Input: part model. Units: mm. Frame: model coordinates. Give positions to 0.01 mm unless a question says otherwise; leave off trailing zeros. Loops run counter-clockwise (first coordinate to the right, second up) from the corner with the lowest first, then second, coordinate; pieces in that order, holes last. Notation, with made-up numbers: (45.5, 47) - (95.5, 47) arc R20 ccw to (95.5, 86) - close; hole circle Ø7 at (58, -34). An arc over 180 degrees is marked (long way). Answer as a JSON object with one key per item and string values.
from build123d import *

# Parameters (mm, degrees)
SKETCH1_R      = 0.6604
EXTRUDE1_DEPTH = 0.5334
FILLET1_R      = 1.1684


with BuildPart() as part:
    # Sketch1 → Extrude1 (new body, symmetric)
    with BuildSketch(Plane(origin=(0, 0, 0), x_dir=(0, 0, -1), z_dir=(1, 0, 0))):
        with BuildLine():
            Line((-0.179532905, 10.28543324), (-0.240263789, 13.76470325))
            Line((-0.240263789, 13.76470325), (-2.849716296, 13.719155087))
            Line((-2.849716296, 13.719155087), (-4.681521945, 10.760524305))
            ThreePointArc((-4.681521945, 10.760524305), (0, -12.9286), (4.681521945, 10.760524305))
            Line((4.681521945, 10.760524305), (2.849716296, 13.719155087))
            Line((2.849716296, 13.719155087), (0.240263789, 13.76470325))
            Line((0.240263789, 13.76470325), (0.179532905, 10.28543324))
            ThreePointArc((0.179532905, 10.28543324), (0, -10.287), (-0.179532905, 10.28543324))
        make_face()
        with Locations((-1.514624601, 12.002294163)):
            Circle(SKETCH1_R, mode=Mode.SUBTRACT)
        with Locations((1.514624601, 12.002294163)):
            Circle(SKETCH1_R, mode=Mode.SUBTRACT)
    extrude(amount=EXTRUDE1_DEPTH, both=True)

    # Fillet1
    fillet1_edges = [part.edges().sort_by_distance(p)[0] for p in [
        (0, 13.719155087, -2.849716296),
        (0, 10.760524305, -4.681521945),
        (0, 10.760524305, 4.681521945),
        (0, 13.719155087, 2.849716296),
    ]]
    fillet(fillet1_edges, radius=FILLET1_R)


solid = part.part
Item 1: Mould query, pull axis Y, two halves, no side actions, for faces 1 (the face through (0.533, -10.4, 1)), 2 (the face through (-0.01, 11.36, 1.66)), 3 (the face through (0.007, 12.14, 3.827)). Classes: released by +Y, released by -Y, zero draft, split by the parting line, or undercut.
Geometry check:
{"face 1": "zero draft", "face 2": "undercut", "face 3": "released by +Y"}
Item 2: Cut plane B-B (z = -1.5). Return loops of the section in (x, y).
Geometry check:
{"outline": "(-0.53, -12.84) - (0.53, -12.84) - (0.53, -10.18) - (-0.53, -10.18) - close; (-0.53, 10.18) - (0.53, 10.18) - (0.53, 11.34) - (-0.53, 11.34) - close; (-0.53, 12.66) - (0.53, 12.66) - (0.53, 13.74) - (-0.53, 13.74) - close"}
Item 3: Cut plane D-D (z = 9.5). Return loops of the section in (x, y), then the cut area to 3 significant figures.
Geometry check:
{"outline": "(-0.53, -8.45) - (0.53, -8.45) - (0.53, -3.95) - (-0.53, -3.95) - close; (-0.53, 3.95) - (0.53, 3.95) - (0.53, 7.2) - (-0.53, 7.2) - close", "area": "8.27 mm2"}
Item 4: Material intervals for line 1 (Y direction, x = 0.5, z = -2) (3 decimals); line 2 (Y direction, x = -0.05, z = 1); line 3 (Z direction, x = -0.05, y = 4.75), sorted ascending. Write a range as [from, to].
Geometry check:
{"line 1": "y = [-12.765, -10.091], [10.091, 11.554], [12.45, 13.734]", "line 2": "y = [-12.89, -10.24], [10.24, 11.59], [12.42, 13.75]", "line 3": "z = [-11.07, -9.12], [9.12, 11.07]"}
Item 5: Cut plane A-A (y = -0.5). Return loops of the section in (x, z), then the cut area to 3 significant figures.
Geometry check:
{"outline": "(-0.53, -12.31) - (0.53, -12.31) - (0.53, -10.27) - (-0.53, -10.27) - close; (-0.53, 10.27) - (0.53, 10.27) - (0.53, 12.31) - (-0.53, 12.31) - close", "area": "4.33 mm2"}
Item 6: Cut plane C-C (x = 0.15). Return loops of the section in (y, z), then the cut area to 3 significant figures.
Geometry check:
{"outline": "(10.29, -0.18) arc R10.29 cw (long way) to (10.29, 0.18) - (13.76, 0.24) - (13.73, 2.21) arc R1.17 ccw to (13.18, 3.19) - (11.07, 4.49) arc R1.17 cw to (10.62, 5.01) arc R12.31 ccw (long way) to (10.62, -5.01) arc R1.17 cw to (11.07, -4.49) - (13.18, -3.19) arc R1.17 ccw to (13.73, -2.21) - (13.76, -0.24) - close; hole circle Ø1.32 at (12, -1.51); hole circle Ø1.32 at (12, 1.51)", "area": "156 mm2"}
